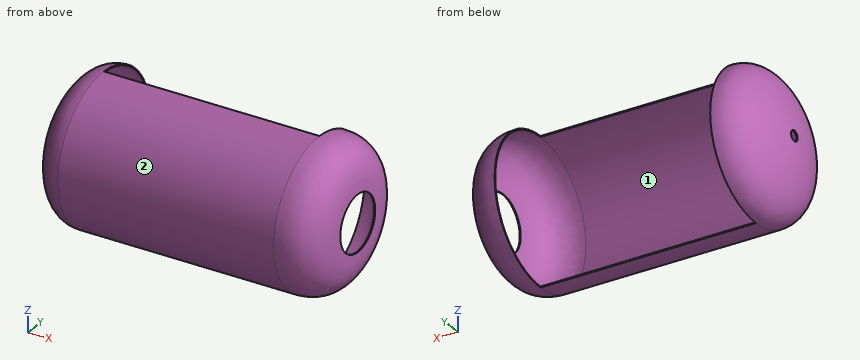
from build123d import *

# Parameters (mm, degrees)
SKETCH4_W          = 958.607886296
SKETCH4_H          = 357.948466727
CUT_EXTRUDE2_DEPTH = 620


with BuildPart() as part:
    # Sketch1 → Revolve1 (revolve)
    with BuildSketch(Plane(origin=(0, 0, 0), x_dir=(1, 0, 0), z_dir=(0, 1, 0))):
        with BuildLine():
            Line((-38.416122965, -102.435963202), (581.583877035, -102.435963202))
            add(Edge.make_bspline(
                [(581.583877035, -102.435963202), (693.455539681, -103.300064727), (691.583877035, -210.80239754), (691.583877035, -232.435963192)],
                knots=[0, 0, 0, 0, 1, 1, 1, 1], degree=3))
            Line((691.583877035, -232.435963192), (688.583877035, -232.435963192))
            add(Edge.make_bspline(
                [(581.572240946, -105.435963202), (582.424150652, -105.442600659), (584.137918536, -105.468851395), (587.484086921, -105.571526796), (591.571096113, -105.792916991), (596.307608869, -106.20262694), (602.409126826, -106.934758126), (609.639419087, -108.18665603), (617.705857071, -110.190510236), (625.186745256, -112.659295822), (634.414245375, -116.523312816), (644.612073728, -122.339029978), (654.913796392, -130.630357057), (663.469285855, -139.982021209), (670.450391217, -150.141502012), (676.016737994, -160.847618745), (680.323342136, -171.829037867), (683.525745861, -182.806951112), (685.782094183, -193.498408861), (687.253383878, -203.618874424), (687.961369137, -211.339785332), (688.299442483, -216.947462036), (688.459593049, -220.834002423), (688.547117141, -224.365875375), (688.582824389, -227.512914091), (688.58674237, -229.777140481), (688.584795317, -231.383827189), (688.583877035, -232.075985649), (688.583877035, -232.435963192)],
                knots=[3.4973e-05, 3.4973e-05, 3.4973e-05, 3.4973e-05, 0.0078472, 0.015659426, 0.03128388, 0.046908334, 0.062532787, 0.093781694, 0.125030601, 0.156279508, 0.187528415, 0.25002623, 0.312524044, 0.375021858, 0.437519672, 0.500017486, 0.562515301, 0.625013115, 0.687510929, 0.750008743, 0.812506557, 0.843755465, 0.875004372, 0.906253279, 0.937502186, 0.968751093, 0.984375546, 1, 1, 1, 1], degree=3))
            Line((581.572240946, -105.435963202), (-38.416122951, -105.435969803))
            add(Edge.make_bspline(
                [(-145.416150087, -297.448719694), (-145.415786094, -297.363118797), (-145.414261278, -297.209117302), (-145.406482156, -296.763589127), (-145.387577621, -296.059017238), (-145.348080967, -294.963719442), (-145.270536885, -293.196191663), (-145.12221169, -290.430217628), (-144.846888777, -286.292241124), (-144.459106758, -281.402026013), (-143.771963774, -273.967299792), (-142.556325425, -263.124157442), (-140.406308296, -248.159348272), (-137.445210779, -231.767940973), (-133.55430361, -214.477141353), (-128.616651259, -196.81526366), (-122.518262583, -179.311948455), (-115.149922932, -162.497881736), (-106.409989847, -146.903194531), (-96.207058742, -133.05233616), (-86.417989624, -123.386032183), (-77.769632288, -117.014146282), (-70.859172034, -112.970513688), (-63.504748075, -109.716446776), (-56.985343251, -107.708604585), (-51.52041341, -106.554160283), (-47.294097057, -105.922162765), (-43.659473987, -105.597170774), (-40.689467236, -105.462466746), (-39.171234927, -105.437583269), (-38.416122951, -105.435969803)],
                knots=[2.115e-05, 2.115e-05, 2.115e-05, 2.115e-05, 0.007833485, 0.015645819, 0.031270489, 0.046895159, 0.062519828, 0.093769167, 0.125018506, 0.156267845, 0.187517184, 0.250015862, 0.312514541, 0.375013219, 0.437511897, 0.500010575, 0.562509253, 0.625007931, 0.687506609, 0.750005287, 0.812503966, 0.843753305, 0.875002644, 0.906251983, 0.937501322, 0.953125991, 0.968750661, 0.98437533, 0.992187665, 1, 1, 1, 1], degree=3))
            Line((-145.416150087, -297.448719694), (-148.416122965, -297.435963202))
            add(Edge.make_bspline(
                [(-38.416122965, -102.435963202), (-139.444928363, -102.64405425), (-148.369931417, -286.57299354), (-148.416122965, -297.435963202)],
                knots=[0, 0, 0, 0, 1, 1, 1, 1], degree=3))
        make_face()
    revolve(axis=Axis((-396.592099756, 0, 312.435963202), (1, 0, 0)))

    # Sketch4 → Cut-Extrude2 (cut)
    with BuildSketch(Plane(origin=(-38.416122965, 0, 0), x_dir=(0, 0, -1), z_dir=(1, 0, 0))):
        with Locations((-258.191988159, 178.974233364)):
            Rectangle(SKETCH4_W, SKETCH4_H)
    extrude(amount=CUT_EXTRUDE2_DEPTH, mode=Mode.SUBTRACT)


solid = part.part
Here's how the part is built. I have some questions about the finished solid (model axes, mm). Face numbers are marked on the shaded views. Round coordinates to 2 decimals unless told otherwise and drop trailing zeros. Order: outer loops, then holes, each group sorted by start corner. A loop starts at its lowest first (then second) coordinate and runs counter-clockwise, first axis right, second up. Notation, with made-up numbers: M 87.5,-29 L 143.5,-29 A17 ccw 143.5,-19 Z; hole C 43,-24.5 d2. An arc over 180 degrees is marked long. Return JSON: item names as keys, results as strings. Group by question number.
1. Please list where these lines run through material, in increasing order: probe 1 along X at (y, z) = (98, 339.5); probe 2 along Z at (x, y) = (323.5, -65.5); probe 3 along X at (y, z) = (-39, 430).
2. If we section it at A-A on x = 509: List the corners of the cut face in (y, z) for me, then the cut area to 3 significant figures.
3. I'm going to push flat-ended pins straight in: pin 1 Ø1.5 at (x, z) = (399, 104.5) entering from +Y; pin 2 Ø6 at (y, z) = (56.5, 269) entering from +X; pin 3 Ø4 at (x, y) = (595.5, -161) entering from -Z. Where does each tip first touch, or does it pass through?
4. If we mould it in two halves opening along X, with no side actions, what happens to the marked faces 1 and 2? For each: pulls with the +X half, pulls with the -X half, needs draft (parallel to the pull), parting line crosses it, or undercut.
Reply:
{
 "1": {"probe 1": "-135.54 to -132.44, 687.88 to 690.89", "probe 2": "112.91 to 116.07, 508.8 to 511.96", "probe 3": "-128.86 to -125.69, 684.71 to 687.78"},
 "2": {"outline": "M 0,102.44 L 0,105.44 A207 cw 0,519.44 L 0,522.44 A210 ccw Z", "area": "1,970 mm^2"},
 "3": {"pin 1": "y = 0", "pin 2": "x = -138.57", "pin 3": "z = 176.31"},
 "4": {"face 1": "undercut", "face 2": "needs draft"}
}
